from build123d import *

# Parameters (mm, degrees)
F1_DEPTH = 63.5
F2_DEPTH = 25.4


with BuildPart() as f1:
    # F0 (on Front) → F1 (new body, symmetric)
    with BuildSketch(Plane.XZ):
        Polygon((-47.625, 9.525), (-47.625, -9.525), (47.625, -9.525), (47.625, 9.525), (28.575, 9.525), align=None)
    extrude(amount=F1_DEPTH, both=True)

    # F0 (on Front) → F2 (join, symmetric)
    with BuildSketch(Plane.XZ):
        Polygon((-47.625, 9.525), (-47.625, -9.525), (47.625, -9.525), (47.625, 9.525), (28.575, 9.525), align=None)
        with BuildLine():
            add(Edge.make_bspline(
                [(-47.625, 9.525), (-46.467692, 38.43854), (24.964292, 61.567295), (58.792322, 61.9252)],
                knots=[0, 0, 0, 0, 118.618833, 118.618833, 118.618833, 118.618833], degree=3))
            Line((-47.625, 9.525), (28.575, 9.525))
            Line((28.575, 9.525), (28.575, 27.318938))
            ThreePointArc((28.575, 27.318938), (37.19248, 50.290006), (58.792322, 61.9252))
        make_face()
        with BuildLine():
            Line((28.575, 9.525), (47.625, 9.525))
            Line((47.625, 9.525), (47.625, 27.318938))
            ThreePointArc((47.625, 27.318938), (51.20645, 37.363053), (60.334826, 42.8752))
            Line((60.334826, 42.8752), (68.441236, 42.8752))
            Line((68.441236, 42.8752), (68.441236, 61.9252))
            Line((68.441236, 61.9252), (58.792322, 61.9252))
            ThreePointArc((58.792322, 61.9252), (37.19248, 50.290006), (28.575, 27.318938))
            Line((28.575, 27.318938), (28.575, 9.525))
        make_face()
        Polygon((68.441236, 66.675), (68.441236, 61.9252), (68.441236, 42.8752), (68.441236, 38.1), (119.241236, 38.1), (119.241236, 66.675), align=None)
    extrude(amount=F2_DEPTH, both=True)


solid = f1.part
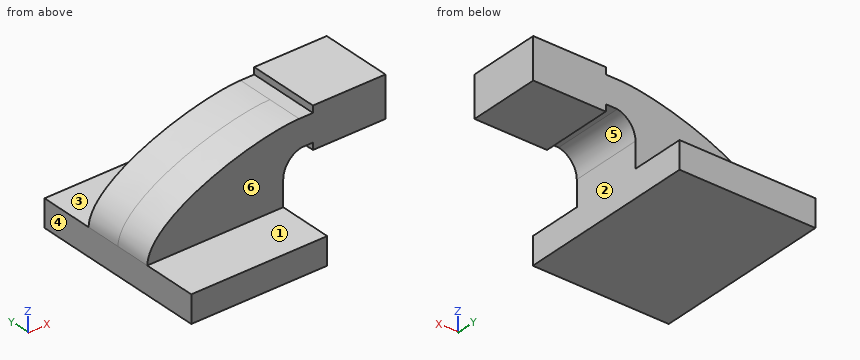
Verification items for the finished model (mm, model axes). Face numbers are marked on the shaded views. A direction names the side the tool comes from. Coordinates: 2 decimals unless noted, no trailing zeros. Order: outer loops, then holes, each group sorted by start corner. A loop starts at its lowest first (then second) coordinate and runs counter-clockwise, first axis right, second up. Notation, with made-up numbers: M 89.5,-19.5 L 145.5,-19.5 A13 ccw 145.5,-11.5 Z; hole C 88,63.25 d5. An arc over 180 degrees is marked long. One line per item, written item: value. Start each with the question number.
Item 1: Depth check by flat-ended pin: P1, Ø1.5, axis at x = 14.5, y = 31.5, coming from the +Z side (3 decimals); P2, Ø1, axis at x = 5, z = 49, coming from the -Y side; P3, Ø7.5, axis at x = 63.5, y = 6, coming from the +Z side. Enter the tip coordinate at first touch or a pass-through.
Item 2: Sectioned sample at A-A on y = 40. Record the cut outline in (x, z) (3 decimals).
Item 3: Mould release check, pull along X, two halves, no side actions. Record for the marked faces 4, 5 and 6: pulls with the +X half, pulls with the -X half, needs draft (parallel to the pull), parting line crosses it, or undercut.
Item 4: Sectioned sample at B-B on x = 64. Record the cut outline in (y, z), then the cut area to 3 significant figures.
Item 5: Access from +Z, -Z, +X, -X, +Y, -Y to the whole of each face (thin tool, end or side, straight path). Record for the marked faces 1, 2 and 3.
Item 6: Thickness scan on probe 1 along Y at (x, z) = (69.5, 56.5); probe 2 along Z at (x, y) = (-31.5, 55.5) (3 decimals); probe 3 along X at (y, z) = (10, 39). Record the ranges inside material, lowest first.
Calculated:
1. P1: z = 9.525
1. P2: y = -25.4
1. P3: z = 61.93
2. outline: M -47.625,-9.525 L 47.625,-9.525 L 47.625,9.525 L -47.625,9.525 Z
3. face 4: pulls with the -X half
3. face 5: undercut
3. face 6: needs draft
4. outline: M -25.4,42.88 L 25.4,42.88 L 25.4,61.93 L -25.4,61.93 Z
4. area: 968 mm^2
5. face 1: +Z, +X, -X, -Y
5. face 2: -Z, +X, +Y, -Y
5. face 3: +Z, +X, -X, +Y
6. probe 1: -25.4 to 25.4
6. probe 2: -9.525 to 9.525
6. probe 3: -21.87 to 52.75, 68.44 to 119.24
